Autodesk Inventor part; units mm, degrees
ref_plane "YZ Plane" through (0, 0, 0) normal (1, 0, 0) x (0, 1, 0)
ref_plane "XZ Plane" through (0, 0, 0) normal (0, 1, 0) x (-1, 0, 0)
ref_plane "XY Plane" through (0, 0, 0) normal (0, 0, 1) x (1, 0, 0)
sketch "スケッチ1" plane through (0, 0, 0) normal (0, 0, 1) x (1, 0, 0)
  circle A0 centre (0, 0) radius 2.75
  dimension "d0" = 5.5
extrude "押し出し1" add sketch "スケッチ1" along normal blind 2.9
sketch "スケッチ2" plane through (0, 0, 0) normal (0, 0, -1) x (-1, 0, 0)
  circle A0 centre (0, 0) radius 1.5
  dimension "d3" = 3
extrude "押し出し2" add sketch "スケッチ2" along normal blind 4
chamfer "面取り1" distance 0.1 angle 45 1 edges at (-2.75, 0, 2.9)
thread "ねじ2"
properties part number "M3×8" material "ステンレス鋼"
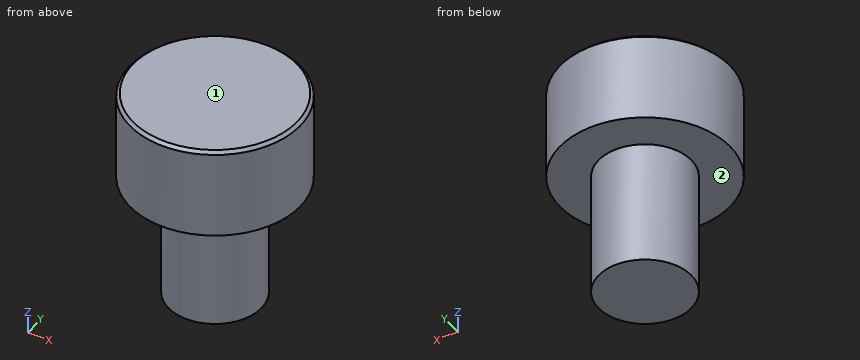
CAD build for the part. Positions are in the model's coordinates, mm. Face numbers are marked on the shaded views. A direction names the side the tool comes from. Give positions to 0.01 mm unless a question says otherwise; leave off trailing zeros. Loops run counter-clockwise (first coordinate to the right, second up) from the corner with the lowest first, then second, coordinate; pieces in that order, holes last. Notation, with made-up numbers: M 3,10 L 54,10 A21 cw 54,28 Z; hole C 8.5,40 d11. An arc over 180 degrees is marked long. Use one line per item in the form item = value.
Item 1: Slice it at D-D (z = 0.75). List the corners of the cut face in (x, y), plus the area to 3 significant figures.
Determined:
outline = C 0,0 d5.5
area = 23.8 mm2
Item 2: Drill centre lines: probe 1 along Z at (x, y) = (1.75, -0.2); probe 2 along Y at (x, z) = (-0.9, -3.25); probe 3 along Y at (x, z) = (0.35, -1.5). Where is each one in solid material? Low to high. Write a range as from..to.
Determined:
probe_1 = 0..2.9
probe_2 = -1.2..1.2
probe_3 = -1.46..1.46
Item 3: Flat gauge pin, fed straight in: pin 1 (1.5 mm diameter, centred on y = -2, z = -1, fed in from -X). Where does the tip first touch, or does it go through?
Determined:
pin_1 = -0.83
Item 4: Slice it at A-A (x = 0). List the corners of the cut face in (y, z).
Determined:
outline = M -2.75,0 L -1.5,0 L -1.5,-4 L 1.5,-4 L 1.5,0 L 2.75,0 L 2.75,2.8 L 2.65,2.9 L -2.65,2.9 L -2.75,2.8 Z
Item 5: Slice it at C-C (z = -0.25). List the corners of the cut face in (x, y).
Determined:
outline = C 0,0 d3
Item 6: Which spindle directions (+Z, -Z, +X, -X, +Y, -Y) get a long thin tool onto all of the face, cutting with end or side? Do the marked faces 1 and 2. Say none if no direction does.
Determined:
face_1 = +Z, +X, -X, +Y, -Y
face_2 = -Z
